Source: CAD feature listing. Evaluate the final solid. Frame: model axes, mm. A direction names the side the tool comes from. Coordinates: 2 decimals unless noted, no trailing zeros. Write each loop counter-clockwise with the first axis right and the second up, starting at its lowest first coordinate (ties: lowest second). Pieces come first, ordered by that corner, then holes. Notation, with made-up numbers: (-4.75, -40) -> (44.25, -40) arc R23 ccw to (44.25, -30) -> close; hole circle Ø7 at (64, 70). An arc over 180 degrees is marked (long way). Write item = value, one per line.
from build123d import *

# Parameters (mm, degrees)
F0_R     = 12.7
F1_DEPTH = 38.1
F2_R     = 6.35
F3_R     = 6.35
F4_DEPTH = 12.7


with BuildPart() as f1:
    # F0 (on Front) → F1 (new body)
    with BuildSketch(Plane.XZ):
        with BuildLine():
            Line((-127, 0), (0, 0))
            Line((0, 0), (0, 12.7))
            Line((0, 12.7), (-31.75, 12.7))
            ThreePointArc((-31.75, 12.7), (-40.908636, 16.60174), (-44.439774, 25.909547))
            ThreePointArc((-44.439774, 25.909547), (-63.506386, 45.757127), (-82.572999, 25.909547))
            ThreePointArc((-82.572999, 25.909547), (-86.104136, 16.60174), (-95.262773, 12.7))
            Line((-95.262773, 12.7), (-127, 12.7))
            Line((-127, 12.7), (-127, 0))
        make_face()
        with Locations((-63.506386, 26.67515)):
            Circle(F0_R, mode=Mode.SUBTRACT)
    extrude(amount=-F1_DEPTH)

    # F2 (on face) + F3 (on face) → F4 (cut)
    with BuildSketch(Plane.XY.offset(12.7)):
        with Locations((-19.05, 19.05)):
            Circle(F2_R)
    with BuildSketch(Plane.XY.offset(12.7)):
        with Locations((-107.95, 19.05)):
            Circle(F3_R)
    extrude(amount=-F4_DEPTH, mode=Mode.SUBTRACT)


solid = f1.part
1) Material intervals for probe 1 along X at (y, z) = (19, 6); probe 2 along X at (y, z) = (16, 3); probe 3 along Y at (x, z) = (-19.05, 8.25), sorted ascending. Write a range as [from, to].
Answer block:
probe_1 = [-127, -114.3], [-101.6, -25.4], [-12.7, 0]
probe_2 = [-127, -113.52], [-102.38, -24.62], [-13.48, 0]
probe_3 = [0, 12.7], [25.4, 38.1]
2) Cut plane B-B, the plane y = 17. Output: boundary loops of the cut face in (x, z).
Answer block:
outline = (-127, 0) -> (-113.96, 0) -> (-113.96, 12.7) -> (-127, 12.7) -> close; (-101.94, 0) -> (-25.06, 0) -> (-25.06, 12.7) -> (-31.75, 12.7) arc R12.7 cw to (-44.44, 25.91) arc R19.08 ccw (long way) to (-82.57, 25.91) arc R12.7 cw to (-95.26, 12.7) -> (-101.94, 12.7) -> close; (-13.04, 0) -> (0, 0) -> (0, 12.7) -> (-13.04, 12.7) -> close; hole circle Ø25.4 at (-63.51, 26.68)
3) Cut plane A-A, the plane x = -19.05. Output: boundary loops of the cut face in (y, z), and give its area (3 significant figures).
Answer block:
outline = (0, 0) -> (12.7, 0) -> (12.7, 12.7) -> (0, 12.7) -> close; (25.4, 0) -> (38.1, 0) -> (38.1, 12.7) -> (25.4, 12.7) -> close
area = 323 mm2
4) First-contact query: pin 1 Ø11.5 at (x, y) = (-107.95, 19.05) entering from +Z; pin 2 Ø9.5 at (x, y) = (-9, 24) entering from +Z; pin 3 Ø5 at (y, z) = (30.5, 38) entering from -X; pin 4 Ø10 at (y, z) = (13, 23.5) entering from -X. Flat tips, straight axial feed; report the tip coordinate or a pass-through.
Answer block:
pin_1 = through
pin_2 = 12.7
pin_3 = -80.43
pin_4 = -84.6
5) Cut plane C-C, the plane z = 37.5. Output: boundary loops of the cut face in (x, y).
Answer block:
outline = (-79.22, 0) -> (-70.15, 0) -> (-70.15, 38.1) -> (-79.22, 38.1) -> close; (-56.86, 0) -> (-47.79, 0) -> (-47.79, 38.1) -> (-56.86, 38.1) -> close
6) Pull-direction query (Y, two-part tool) for faces 1 (the cylindrical face through (-19.877, 25.346, 6.439)), 2 (the flat face through (-64, 19, 0)), 3 (the flat face through (-64, 38.1, 13)); classes: +Y half, -Y half, draft (parallel to the pull), parting line (faces both ways), or undercut.
Answer block:
face_1 = undercut
face_2 = draft
face_3 = +Y half
7) Cut plane D-D, the plane y = 10.5. Output: boundary loops of the cut face in (x, z).
Answer block:
outline = (-127, 0) -> (0, 0) -> (0, 12.7) -> (-31.75, 12.7) arc R12.7 cw to (-44.44, 25.91) arc R19.08 ccw (long way) to (-82.57, 25.91) arc R12.7 cw to (-95.26, 12.7) -> (-127, 12.7) -> close; hole circle Ø25.4 at (-63.51, 26.68)
8) Reachability of faces 4 (the flat face through (-12, 19, 12.7)), 5 (the cylindrical face through (-65.16, 18.783, 39.267)), 6 (the flat face through (-114, 23, 12.7)) from +Z, -Z, +X, -X, +Y, -Y: full face, straight path, thin tool, end or side. Return the list, or none.
Answer block:
face_4 = +Z, +X, +Y, -Y
face_5 = +Y, -Y
face_6 = +Z, -X, +Y, -Y
